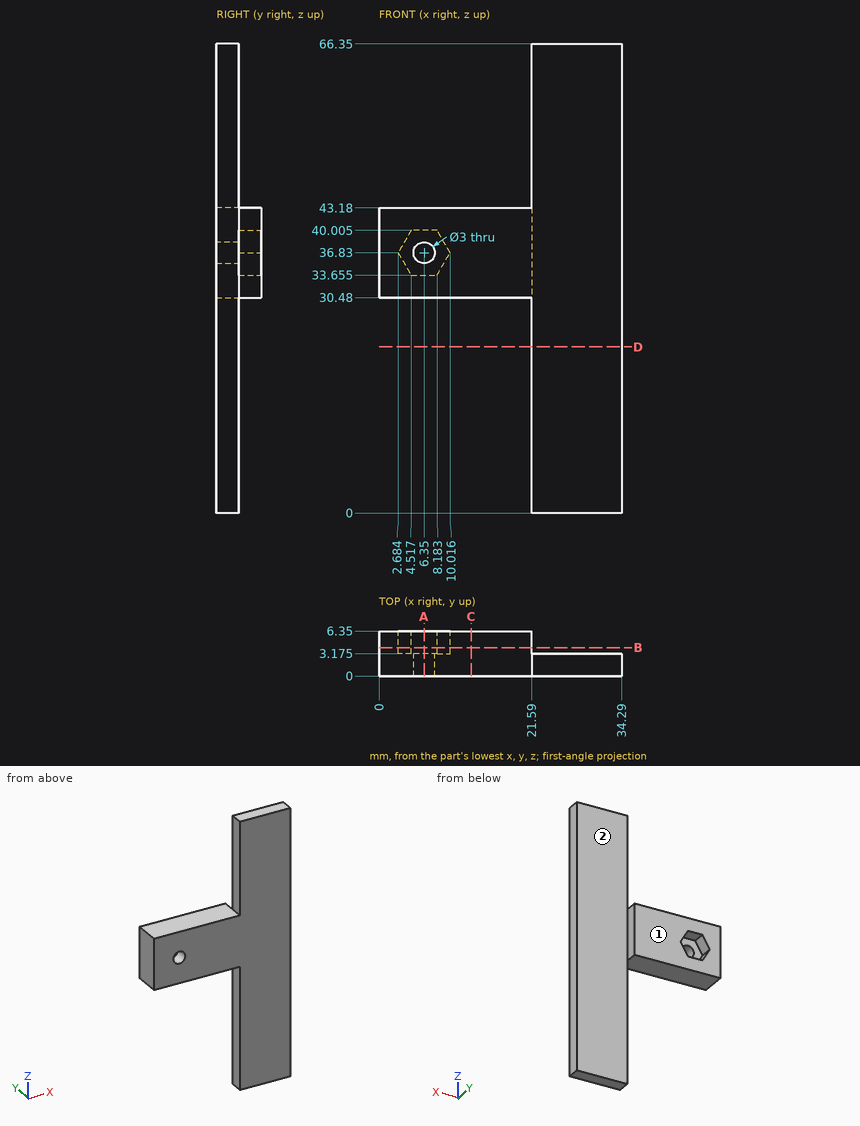
Here's the drawing with two shaded views (mm, measured from the low corner). I have some questions. A direction names the side the tool comes from. Coordinates: 2 decimals unless noted, no trailing zeros. Order: outer loops, then holes, each group sorted by start corner. A loop starts at its lowest first (then second) coordinate and runs counter-clockwise, first axis right, second up. Notation, with made-up numbers: (-5, -27) - (43, -27) arc R6 cw to (43, -16) - close; hole circle Ø11 at (24, 31.25). An arc over 180 degrees is marked (long way). Use CSV: the item, a comma, the result in double quotes. Start each with the question number.
1. I'm going to push flat-ended pins straight in: pin 1 (1 mm diameter, centred on y = 1.5, z = 55.5, fed in from -X); pin 2 (3 mm diameter, centred on x = 11, y = 2, fed in from +Z); pin 3 (6 mm diameter, centred on x = 20.5, z = 26.5, fed in from +Y) (3 decimals). Where does each tip first touch, or does it pass through?
2. Suppose I cut it at C-C on x = 13. List the corners of the cut face in (y, z) for me.
3. Please list where these lines run through material, in increasing order: line 1 (X direction, y = 1, z = 36.83); line 2 (Z direction, x = 8, y = 5.5) (3 decimals); line 3 (Y direction, x = 24, z = 63) (3 decimals). Write a range as from..to.
4. Suppose I cut it at D-D on z = 23.5. List the corners of the cut face in (x, y) for me (3 decimals), then the cut area to 3 significant figures.
5. Suppose I cut it at B-B on y = 4. List the corners of the cut face in (x, z) for me (1 decimal), then the cut area to 3 significant figures.
6. For the marked faces 1 and 2, which set-ups out of +Z, -Z, +X, -X, +Y, -Y let a thin tool reach every point of the face, with its end or its side?
7. Suppose I cut it at A-A on x = 6.35. List the corners of the cut face in (y, z) for me (3 decimals).
Output:
1,pin 1,"stops at x = 21.59"
1,pin 2,"stops at z = 43.18"
1,pin 3,"stops at y = 3.175"
2,outline,"(0, 30.48) - (6.35, 30.48) - (6.35, 43.18) - (0, 43.18) - close"
3,line 1,"x = 0..4.85, 7.85..34.29"
3,line 2,"z = 30.48..33.655, 40.005..43.18"
3,line 3,"y = 0..3.175"
4,outline,"(21.59, 0) - (34.29, 0) - (34.29, 3.175) - (21.59, 3.175) - close"
4,area,"40.3 mm2"
5,outline,"(0, 30.5) - (21.6, 30.5) - (21.6, 43.2) - (0, 43.2) - close; hole (2.7, 36.8) - (4.5, 33.7) - (8.2, 33.7) - (10, 36.8) - (8.2, 40) - (4.5, 40) - close"
5,area,"239 mm2"
6,face 1,"+Z, -Z, +X, -X, +Y"
6,face 2,"+Z, -Z, +X, +Y"
7,outline,"(0, 30.48) - (6.35, 30.48) - (6.35, 33.655) - (3.175, 33.655) - (3.175, 35.33) - (0, 35.33) - close; (0, 38.33) - (3.175, 38.33) - (3.175, 40.005) - (6.35, 40.005) - (6.35, 43.18) - (0, 43.18) - close"
